For this review, take the finished solid that the model builds, in its own axes (mm). Give positions to 0.01 mm unless a question says otherwise; leave off trailing zeros. Order: outer loops, then holes, each group sorted by start corner. A loop starts at its lowest first (then second) coordinate and runs counter-clockwise, first axis right, second up.
Item 1: Consider section B-B (x = -5.5). Give the number of separate pieces and of enclosed holes in the cut face, plus the area to 3 significant figures.
Item 2: For P1, Ø6, axis at x = 0, y = 0, coming from the -Z side, flat-tipped, find the tip position at first contact; note if it passes through.
Item 3: The part is to be moulded in two halves that separate along Y. For faces 1 (the conical face through (-2.4, -25.23, 0.13)), 2 (the flat face through (5, 1, 0.508)), 3 (the conical face through (1.937, 26.156, 0.129)), 4 (the conical face through (25.553, -1.121, 0.383)), say which applies: released by +Y, released by -Y, zero draft, split by the parting line, or undercut.
Item 4: Consider section A-A (z = 0.35). Give the boundary of the cut face in (x, y).
Item 5: For probe 1 along Y at (x, z) = (5, 0.45); probe 2 along Y at (x, z) = (-4.5, 0.1); probe 3 along X at (y, z) = (5.5, 0.3), list the stretches that pass through material, from the lowest coordinate up.
```python
from build123d import *

# Parameters (mm, degrees)
F0_R        = 3.6516934022
F1_DEPTH    = 0.508
F2_C1_SIZE  = 0.254
F2_C2_SIZE  = 0.2539
F2_C3_SIZE  = 0.254
F2_C4_SIZE  = 0.2539
F2_C5_SIZE  = 0.254
F2_C6_SIZE  = 0.2539
F2_C7_SIZE  = 0.254
F2_C8_SIZE  = 0.2539
F2_C9_SIZE  = 0.2539
F2_C10_SIZE = 0.2536
F2_C11_SIZE = 0.254
F2_C12_SIZE = 0.2539
F2_C13_SIZE = 0.2539
F2_C14_SIZE = 0.2536
F2_C15_SIZE = 0.2539
F2_C16_SIZE = 0.2536
F2_C17_SIZE = 0.2539
F2_C18_SIZE = 0.2536


# Not quite as in the source:
# - a fillet or chamfer is up to 0.001 mm smaller than in the source, because OpenCascade refuses the exact size


with BuildPart() as f1:
    # F0 (on Top) → F1 (new body)
    with BuildSketch(Plane.XY):
        with BuildLine():
            ThreePointArc((-4.6809479161, -4.4692134998), (-4.2851428425, -4.9358337251), (-3.9462508024, -5.445292532))
            ThreePointArc((-3.9462508024, -5.445292532), (-3.2543970352, -7.5756381968), (-3.5123975908, -9.8006033651))
            ThreePointArc((-3.5123975908, -9.8006033651), (0.5657181683, -9.1143610896), (4.2157772611, -11.0583325976))
            ThreePointArc((4.2157772611, -11.0583325976), (4.0349146255, -4.7562355253), (10.0331924761, -2.8146378249))
            ThreePointArc((10.0331924761, -2.8146378249), (9.3469502005, 1.2634779342), (11.2909217086, 4.913537027))
            ThreePointArc((11.2909217086, 4.913537027), (7.9764094343, 3.7712610201), (4.6809479161, 4.9673878837))
            ThreePointArc((4.6809479161, 4.9673878837), (4.4188770442, 5.1978976137), (4.1726827472, 5.445292532))
            ThreePointArc((4.1726827472, 5.445292532), (2.8785820733, 7.9323939108), (3.0472269358, 10.730952242))
            ThreePointArc((3.0472269358, 10.730952242), (-1.0308888232, 10.0447099664), (-4.6809479161, 11.9886814745))
            ThreePointArc((-4.6809479161, 11.9886814745), (-4.5000852805, 5.6865844021), (-10.498363131, 3.7449867017))
            ThreePointArc((-10.498363131, 3.7449867017), (-9.8121208555, -0.3331290573), (-11.7560923635, -3.9831881502))
            ThreePointArc((-11.7560923635, -3.9831881502), (-8.1241949781, -2.8530951946), (-4.6809479161, -4.4692134998))
        make_face()
        Circle(F0_R, mode=Mode.SUBTRACT)
        with BuildLine():
            ThreePointArc((-10.498363131, 3.7449867017), (-26.1092040598, 2.319155388), (-11.7560923635, -3.9831881502))
            ThreePointArc((-11.7560923635, -3.9831881502), (-9.8121208555, -0.3331290573), (-10.498363131, 3.7449867017))
        make_face()
        with BuildLine():
            ThreePointArc((4.2157772611, -11.0583325976), (0.5657181683, -9.1143610896), (-3.5123975908, -9.8006033651))
            ThreePointArc((-3.5123975908, -9.8006033651), (-2.0865662771, -25.4114442939), (4.2157772611, -11.0583325976))
        make_face()
        with BuildLine():
            ThreePointArc((11.2909217086, 4.913537027), (9.3469502005, 1.2634779342), (10.0331924761, -2.8146378249))
            ThreePointArc((10.0331924761, -2.8146378249), (25.6440334048, -1.3888065112), (11.2909217086, 4.913537027))
        make_face()
        with BuildLine():
            ThreePointArc((3.0472269358, 10.730952242), (1.6213956221, 26.3417931707), (-4.6809479161, 11.9886814745))
            ThreePointArc((-4.6809479161, 11.9886814745), (-1.0308888232, 10.0447099664), (3.0472269358, 10.730952242))
        make_face()
    extrude(amount=F1_DEPTH)

    # F2: chamfer of 0.254 on 18 edges, made by hand

    # F2_c1
    f2_c1_edges = [f1.edges().sort_by_distance(p)[0] for p in [
        (-5.4539952912, -3.8023255146, 0),
    ]]
    chamfer(f2_c1_edges, length=F2_C1_SIZE)

    # F2_c2 (size 0.254 in the source; OpenCascade refuses exactly that, so slightly less here)
    f2_c2_edges = [f1.edges().sort_by_distance(p)[0] for p in [
        (-5.4539952912, -3.8023255146, 0.508),
    ]]
    chamfer(f2_c2_edges, length=F2_C2_SIZE)

    # F2_c3
    f2_c3_edges = [f1.edges().sort_by_distance(p)[0] for p in [
        (4.0349146255, -4.7562355253, 0),
    ]]
    chamfer(f2_c3_edges, length=F2_C3_SIZE)

    # F2_c4 (size 0.254 in the source; OpenCascade refuses exactly that, so slightly less here)
    f2_c4_edges = [f1.edges().sort_by_distance(p)[0] for p in [
        (4.0349146255, -4.7562355253, 0.508),
    ]]
    chamfer(f2_c4_edges, length=F2_C4_SIZE)

    # F2_c5
    f2_c5_edges = [f1.edges().sort_by_distance(p)[0] for p in [
        (4.9888246362, 4.7326743914, 0),
    ]]
    chamfer(f2_c5_edges, length=F2_C5_SIZE)

    # F2_c6 (size 0.254 in the source; OpenCascade refuses exactly that, so slightly less here)
    f2_c6_edges = [f1.edges().sort_by_distance(p)[0] for p in [
        (4.9888246362, 4.7326743914, 0.508),
    ]]
    chamfer(f2_c6_edges, length=F2_C6_SIZE)

    # F2_c7
    f2_c7_edges = [f1.edges().sort_by_distance(p)[0] for p in [
        (-4.5000852805, 5.6865844021, 0),
    ]]
    chamfer(f2_c7_edges, length=F2_C7_SIZE)

    # F2_c8 (size 0.254 in the source; OpenCascade refuses exactly that, so slightly less here)
    f2_c8_edges = [f1.edges().sort_by_distance(p)[0] for p in [
        (-4.5000852805, 5.6865844021, 0.508),
    ]]
    chamfer(f2_c8_edges, length=F2_C8_SIZE)

    # F2_c9 (size 0.254 in the source; OpenCascade refuses exactly that, so slightly less here)
    f2_c9_edges = [f1.edges().sort_by_distance(p)[0] for p in [
        (-26.1092040598, 2.319155388, 0),
    ]]
    chamfer(f2_c9_edges, length=F2_C9_SIZE)

    # F2_c10 (size 0.254 in the source; OpenCascade refuses exactly that, so slightly less here)
    f2_c10_edges = [f1.edges().sort_by_distance(p)[0] for p in [
        (-26.1092040598, 2.319155388, 0.508),
    ]]
    chamfer(f2_c10_edges, length=F2_C10_SIZE)

    # F2_c11
    f2_c11_edges = [f1.edges().sort_by_distance(p)[0] for p in [
        (-3.6516934022, 0, 0),
    ]]
    chamfer(f2_c11_edges, length=F2_C11_SIZE)

    # F2_c12 (size 0.254 in the source; OpenCascade refuses exactly that, so slightly less here)
    f2_c12_edges = [f1.edges().sort_by_distance(p)[0] for p in [
        (-3.6516934022, 0, 0.508),
    ]]
    chamfer(f2_c12_edges, length=F2_C12_SIZE)

    # F2_c13 (size 0.254 in the source; OpenCascade refuses exactly that, so slightly less here)
    f2_c13_edges = [f1.edges().sort_by_distance(p)[0] for p in [
        (-2.0865662771, -25.4114442939, 0),
    ]]
    chamfer(f2_c13_edges, length=F2_C13_SIZE)

    # F2_c14 (size 0.254 in the source; OpenCascade refuses exactly that, so slightly less here)
    f2_c14_edges = [f1.edges().sort_by_distance(p)[0] for p in [
        (-2.0865662771, -25.4114442939, 0.508),
    ]]
    chamfer(f2_c14_edges, length=F2_C14_SIZE)

    # F2_c15 (size 0.254 in the source; OpenCascade refuses exactly that, so slightly less here)
    f2_c15_edges = [f1.edges().sort_by_distance(p)[0] for p in [
        (25.6440334048, -1.3888065112, 0),
    ]]
    chamfer(f2_c15_edges, length=F2_C15_SIZE)

    # F2_c16 (size 0.254 in the source; OpenCascade refuses exactly that, so slightly less here)
    f2_c16_edges = [f1.edges().sort_by_distance(p)[0] for p in [
        (25.6440334048, -1.3888065112, 0.508),
    ]]
    chamfer(f2_c16_edges, length=F2_C16_SIZE)

    # F2_c17 (size 0.254 in the source; OpenCascade refuses exactly that, so slightly less here)
    f2_c17_edges = [f1.edges().sort_by_distance(p)[0] for p in [
        (1.6213956221, 26.3417931707, 0),
    ]]
    chamfer(f2_c17_edges, length=F2_C17_SIZE)

    # F2_c18 (size 0.254 in the source; OpenCascade refuses exactly that, so slightly less here)
    f2_c18_edges = [f1.edges().sort_by_distance(p)[0] for p in [
        (1.6213956221, 26.3417931707, 0.508),
    ]]
    chamfer(f2_c18_edges, length=F2_C18_SIZE)


solid = f1.part
```
Resolved:
1. separate pieces: 3
1. enclosed holes: 0
1. area: 16.2 mm2
2. P1: passes through
3. face 1: undercut
3. face 2: zero draft
3. face 3: undercut
3. face 4: split by the parting line
4. outline: (-11.82, -3.91) arc R5.35 cw to (-3.44, -9.88) arc R8 ccw (long way) to (4.15, -11.13) arc R5.35 cw to (10.11, -2.74) arc R8 ccw (long way) to (11.36, 4.84) arc R5.35 cw to (2.97, 10.81) arc R8 ccw (long way) to (-4.61, 12.06) arc R5.35 cw to (-10.57, 3.67) arc R8 ccw (long way) to start; hole circle Ø7.5 at (0, 0)
5. probe 1: y = -22.8 to -12.05, -3.47 to 4.49, 11.99 to 24.72
5. probe 2: y = -24.44 to -10.4, -4.44 to 5.43, 12.01 to 24.66
5. probe 3: x = -24.81 to -11.43, -4.58 to 4.06, 11.86 to 23.45
